```python
from build123d import *

# Parameters (mm, degrees)
SKETCH1_R               = 5
SKETCH1_R_2             = 2.5
BOSS_EXTRUDE1_DEPTH     = 20
CUT_EXTRUDE1_DEPTH      = 73.947048844
CUT_EXTRUDE1_DEPTH_BACK = 73.947048844
CUT_EXTRUDE2_DEPTH      = 87.382039929
CUT_EXTRUDE2_DEPTH_BACK = 87.382039929
CUT_EXTRUDE3_DEPTH      = 67.708320321
CIRPATTERN1_COUNT       = 2
CIRPATTERN1_ANGLE       = 90


with BuildPart() as part:
    # Sketch1 → Boss-Extrude1 (new body)
    with BuildSketch(Plane(origin=(0, 0, 0), x_dir=(1, 0, 0), z_dir=(0, 1, 0))):
        with BuildLine():
            Line((-41.25, -4.841229183), (-3.75, -14.523687548))
            ThreePointArc((-3.75, -14.523687548), (10.606601718, -10.606601718), (14.523687548, 3.75))
            Line((14.523687548, 3.75), (4.841229183, 41.25))
            ThreePointArc((4.841229183, 41.25), (-0.014355404, 44.999979392), (-4.848327042, 41.222180386))
            Line((-4.848327042, 41.222180386), (-10.709838692, 17.969863651))
            ThreePointArc((-10.709838692, 17.969863651), (-13.330617196, 13.456564929), (-17.868360534, 10.878342533))
            Line((-17.868360534, 10.878342533), (-41.25, 4.841229183))
            ThreePointArc((-41.25, 4.841229183), (-45, 0), (-41.25, -4.841229183))
        make_face()
        with Locations(Location((0, 0, 0), (0, 0, 270))):
            Circle(SKETCH1_R, mode=Mode.SUBTRACT)
        with Locations(Location((0, 40, 0), (0, 0, 270))):
            Circle(SKETCH1_R_2, mode=Mode.SUBTRACT)
        with Locations(Location((-40, 0, 0), (0, 0, 270))):
            Circle(SKETCH1_R_2, mode=Mode.SUBTRACT)
    extrude(amount=BOSS_EXTRUDE1_DEPTH)

    # 3DSketch4 → Cut-Extrude1 (cut, two sides)
    with BuildSketch(Plane(origin=(0, 16.470335, -40), x_dir=(0, -0.36901261681753356, 0.9294243856438652), z_dir=(1, 0, 0))) as cut_extrude1_sk:
        with BuildLine():
            Line((0, 0), (13.941365785, -5.535189252))
            ThreePointArc((13.941365785, -5.535189252), (17.767783679, -5.478735371), (20.433550797, -2.733130408))
            Line((20.433550797, -2.733130408), (21.518695129, 0))
            ThreePointArc((21.518695129, 0), (21.462241248, 3.826417894), (18.716636285, 6.492185012))
            Line((18.716636285, 6.492185012), (4.7752705, 12.027374265))
            Line((4.7752705, 12.027374265), (-8.558795166, 17.321445025))
            Line((-8.558795166, 17.321445025), (-13.334065667, 5.294070761))
            Line((-13.334065667, 5.294070761), (0, 0))
        make_face()
    extrude(amount=CUT_EXTRUDE1_DEPTH, mode=Mode.SUBTRACT)
    extrude(cut_extrude1_sk.sketch, amount=-CUT_EXTRUDE1_DEPTH_BACK, mode=Mode.SUBTRACT)

    # 3DSketch5 → Cut-Extrude2 (cut, two sides)
    with BuildSketch(Plane(origin=(-56.872003502, 16.470335, 0), x_dir=(0.9798226496463329, -0.1998688951288811, 0), z_dir=(0, 0, -1))) as cut_extrude2_sk:
        with BuildLine():
            Line((0, 0), (33.243187397, -6.781103844))
            ThreePointArc((33.243187397, -6.781103844), (37.000084817, -6.052830051), (39.141645121, -2.881335071))
            Line((39.141645121, -2.881335071), (39.729393585, 0))
            ThreePointArc((39.729393585, 0), (39.001119792, 3.75689742), (35.829624813, 5.898457724))
            Line((35.829624813, 5.898457724), (2.586437415, 12.679561568))
            Line((2.586437415, 12.679561568), (0, 0))
        make_face()
    extrude(amount=CUT_EXTRUDE2_DEPTH, mode=Mode.SUBTRACT)
    extrude(cut_extrude2_sk.sketch, amount=-CUT_EXTRUDE2_DEPTH_BACK, mode=Mode.SUBTRACT)

    # Sketch2 → Cut-Extrude3 (cut, through all)
    with BuildSketch(Plane(origin=(0, 20, 0), x_dir=(1, 0, 0), z_dir=(0, 1, 0))):
        with BuildLine():
            Line((-30.589723784, 4.495313989), (-17.164379291, 7.962110305))
            Line((-17.164379291, 7.962110305), (-15.226453583, 8.462536474))
            ThreePointArc((-15.226453583, 8.462536474), (-12.714609551, 7.682081043), (-12.291345207, 5.086061319))
            ThreePointArc((-12.291345207, 5.086061319), (-13.302074527, 0), (-12.291345207, -5.086061319))
            ThreePointArc((-12.291345207, -5.086061319), (-12.714609551, -7.682081043), (-15.226453583, -8.462536474))
            Line((-15.226453583, -8.462536474), (-17.164379291, -7.962110305))
            Line((-17.164379291, -7.962110305), (-30.589723784, -4.495313989))
            Line((-30.589723784, -4.495313989), (-30.829716392, -4.433341241))
            ThreePointArc((-30.829716392, -4.433341241), (-32.325817378, -3.33586596), (-32.653488198, -1.509557665))
            ThreePointArc((-32.653488198, -1.509557665), (-32.5, 0), (-32.653488198, 1.509557665))
            ThreePointArc((-32.653488198, 1.509557665), (-32.325817378, 3.33586596), (-30.829716392, 4.433341241))
            Line((-30.829716392, 4.433341241), (-30.589723784, 4.495313989))
        make_face()
    cut_extrude3 = extrude(amount=-CUT_EXTRUDE3_DEPTH, mode=Mode.SUBTRACT)

    # CirPattern1: Cut-Extrude3 ×2 about axis
    cirpattern1_axis = Axis((0, 0, 0), (0, -1, 0))
    for i in range(1, CIRPATTERN1_COUNT):
        add(cut_extrude3.rotate(cirpattern1_axis, i * CIRPATTERN1_ANGLE / (CIRPATTERN1_COUNT - 1)), mode=Mode.SUBTRACT)


solid = part.part
```
Here's how the part is built. I have some questions about the finished solid (model axes, mm). A direction names the side the tool comes from. Give positions to 0.01 mm unless a question says otherwise; leave off trailing zeros. Loops run counter-clockwise (first coordinate to the right, second up) from the corner with the lowest first, then second, coordinate; pieces in that order, holes last. Notation, with made-up numbers: M 67.25,26 L 125.25,26 A17 ccw 125.25,57 Z; hole C 62.25,30.25 d5. An arc over 180 degrees is marked long. Use one line per item in the form item = value. Start each with the question number.
Q1. Will these pins go through, and if not, where does the flat tip stop? pin 1 Ø3 at (y, z) = (10.5, 9) entering from -X; pin 2 Ø7.5 at (x, z) = (-4, -30) entering from +Y; pin 3 Ø6 at (x, y) = (-19.5, 10.5) entering from +Z; pin 4 Ø5 at (y, z) = (9, -22) entering from +X.
Q2. If we section it at B-B (x = 0): Write out the boundary of the cut face in (y, z).
Q3. If we section it at C-C (y = 13.5): Write out the boundary of the cut face in (x, z), then the cut area to 3 significant figures.
Q4. I need wall thicknesses on line 1 along Y through (x, z) = (-36, 2.5); line 2 along X through (y, z) = (10.5, 0); line 3 along X through (y, z) = (1.35, -40). Which ranges of each line are inside material? Lowest first, please.
Q5. Which directions (+Z, -Z, +X, -X, +Y, -Y) give clear straight access to the entire face, cutting with the end or side of a thin tool? Please do faces 1 (the cylindrical face through (-13.278, 9.86, -13.509)), 2 (the cylindrical face through (-8.1, 15.04, -21.5)), 3 (the cylindrical face through (3.31, 1.79, -32.34)).
Q6. If we section it at A-A (z = 0): Write out the boundary of the cut face in (x, y).
Q7. If we section it at D-D (x = -29): Write out the boundary of the cut face in (y, z).
Q8. Thinking about a two-plate mould opening in Z: for faces 4 (the flat face through (-7.738, 3.193, -29.759)), 5 (the cylindrical face through (-12.74, 10.14, -7.71)), 6 (the flat face through (-34, 3.53, 0)), which applies, +Z half, -Z half, draft (parallel to the pull), parting line (faces both ways), or undercut?
Taken from the geometry:
q1.pin_1 = -17.97
q1.pin_2 = 20
q1.pin_3 = 11.23
q1.pin_4 = 10.46
q2.outline = M 0,-45 L 3.53,-45 L 3.53,-42.5 L 0,-42.5 Z; M 0,-37.5 L 3.53,-37.5 L 3.53,-32.5 L 0,-32.5 Z; M 0,-13.3 L 20,-13.3 L 20,-5 L 0,-5 Z; M 0,5 L 20,5 L 20,15 L 0,15 Z; M 16.47,-45 L 20,-45 L 20,-42.5 L 16.47,-42.5 Z; M 16.47,-37.5 L 20,-37.5 L 20,-32.5 L 16.47,-32.5 Z
q3.outline = M -18.37,-10.75 L -17.87,-10.88 A10 cw -10.71,-17.97 L -10.09,-20.43 L -7.12,-20.43 L -8.46,-15.23 A2.5 cw -5.09,-12.29 A13.3 ccw 5.09,-12.29 A2.5 cw 8.46,-15.23 L 7.12,-20.43 L 10.22,-20.43 L 14.52,-3.75 A15 ccw -3.75,14.52 L -18.37,10.75 L -18.37,7.65 L -15.23,8.46 A2.5 cw -12.29,5.09 A13.3 ccw -12.29,-5.09 A2.5 cw -15.23,-8.46 L -18.37,-7.65 Z; hole C 0,0 d10
q3.area = 703 mm^2
q4.line_1 = 0 to 3.53, 16.47 to 20
q4.line_2 = -13.3 to -5, 5 to 15
q4.line_3 = -5.16 to -2.5, 2.5 to 5.16
q5.face_1 = -Z, -X, +Y, -Y
q5.face_2 = -Z, +X, -X
q5.face_3 = +Y, -Y
q6.outline = M -45,0 L -42.5,0 L -42.5,3.53 L -45,3.53 Z; M -45,16.47 L -42.5,16.47 L -42.5,20 L -45,20 Z; M -37.5,0 L -32.5,0 L -32.5,3.53 L -37.5,3.53 Z; M -37.5,16.47 L -32.5,16.47 L -32.5,20 L -37.5,20 Z; M -13.3,0 L -5,0 L -5,20 L -13.3,20 Z; M 5,0 L 15,0 L 15,20 L 5,20 Z
q7.outline = M 0,-8 L 3.53,-8 L 3.53,-4.91 L 0,-4.91 Z; M 0,4.91 L 3.53,4.91 L 3.53,8 L 0,8 Z; M 16.47,-8 L 20,-8 L 20,-4.91 L 16.47,-4.91 Z; M 16.47,4.91 L 20,4.91 L 20,8 L 16.47,8 Z
q8.face_4 = -Z half
q8.face_5 = undercut
q8.face_6 = draft
